CAD build for the part. Positions are in the model's coordinates, mm. Coordinates: 2 decimals unless noted, no trailing zeros. Order: outer loops, then holes, each group sorted by start corner. A loop starts at its lowest first (then second) coordinate and runs counter-clockwise, first axis right, second up.
from build123d import *

# Parameters (mm, degrees)
BOSS_EXTRUDE1_DEPTH = 222.25
SKETCH5_R           = 6.35
BOSS_EXTRUDE2_DEPTH = 7.9375


with BuildPart() as part:
    # Sketch1 → Boss-Extrude1 (new, symmetric)
    with BuildSketch(Plane.XY):
        with BuildLine():
            ThreePointArc((0.93173274, 6.79441227), (0, 6.858), (-0.93173274, 6.79441227))
            Line((-0.93173274, 6.79441227), (-5.41826726, 4.204110358))
            ThreePointArc((-5.41826726, 4.204110358), (-5.939202219, 3.429), (-6.35, 2.590301913))
            Line((-6.35, 2.590301913), (-6.35, -2.590301913))
            ThreePointArc((-6.35, -2.590301913), (-5.939202219, -3.429), (-5.41826726, -4.204110358))
            Line((-5.41826726, -4.204110358), (-0.93173274, -6.79441227))
            ThreePointArc((-0.93173274, -6.79441227), (0, -6.858), (0.93173274, -6.79441227))
            Line((0.93173274, -6.79441227), (5.41826726, -4.204110358))
            ThreePointArc((5.41826726, -4.204110358), (5.939202219, -3.429), (6.35, -2.590301913))
            Line((6.35, -2.590301913), (6.35, 2.590301913))
            ThreePointArc((6.35, 2.590301913), (5.939202219, 3.429), (5.41826726, 4.204110358))
            Line((5.41826726, 4.204110358), (0.93173274, 6.79441227))
        make_face()
    extrude(amount=BOSS_EXTRUDE1_DEPTH, both=True)

    # Sketch5 → Boss-Extrude2 (add)
    with BuildSketch(Plane.XY.offset(222.25)):
        Circle(SKETCH5_R)
    boss_extrude2 = extrude(amount=BOSS_EXTRUDE2_DEPTH)

    # Sketch6 → #10-32 Tapped Hole2 (revolve, cut)
    with BuildSketch(Plane(origin=(0, 0, 230.1875), x_dir=(0, -1, 0), z_dir=(1, 0, 0))):
        Polygon((0, 0), (0, 16.290757848), (2.0193, 15.07744), (2.0193, 0), align=None)
    f_10_32_tapped_hole2 = revolve(axis=Axis((0, 0, 236.5375), (0, 0, -1)), mode=Mode.SUBTRACT)

    # Mirror1: Boss-Extrude2, #10-32 Tapped Hole2 across plane
    add(boss_extrude2.mirror(Plane.XY))
    add(f_10_32_tapped_hole2.mirror(Plane.XY), mode=Mode.SUBTRACT)


solid = part.part
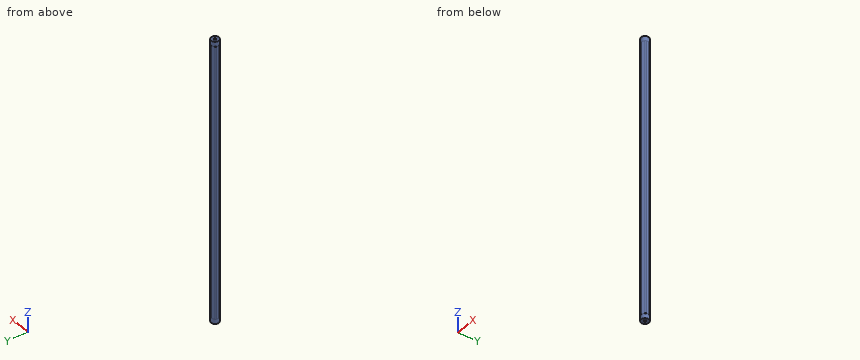
1) Slice it at A-A (z = -166). List the corners of the cut face in (x, y), plus the area to 3 significant figures.
2) Drill centre lines: probe 1 along X at (y, z) = (0, 220.5); probe 2 along Y at (x, z) = (0, -220). Where is each one in solid material? Low to high.
3) Pin check, flat tips, straight feed: P1, Ø4, axis at x = -4, z = -82, coming from the -Y side; P2, Ø1, axis at y = 5.5, z = -150.5, coming from the +X side; P3, Ø1.5, axis at x = 4.5, z = -85, coming from the -Y side. Stop position of each tip, or through.
Worked out:
1. outline: (-6.35, -2.59) arc R6.86 ccw to (-5.42, -4.2) - (-0.93, -6.79) arc R6.86 ccw to (0.93, -6.79) - (5.42, -4.2) arc R6.86 ccw to (6.35, -2.59) - (6.35, 2.59) arc R6.86 ccw to (5.42, 4.2) - (0.93, 6.79) arc R6.86 ccw to (-0.93, 6.79) - (-5.42, 4.2) arc R6.86 ccw to (-6.35, 2.59) - close
1. area: 137 mm2
2. probe 1: x = -6.35 to -2.02, 2.02 to 6.35
2. probe 2: y = -6.86 to -2.02, 2.02 to 6.86
3. P1: stops at y = -6.18
3. P2: stops at x = 4.04
3. P3: stops at y = -5.17
